from build123d import *

# Parameters (mm, degrees)
BOSS_EXTRUDE1_DEPTH = 3
BOSS_EXTRUDE2_DEPTH = 0.63
FILLET1_R           = 0.5


with BuildPart() as part:
    # Sketch1 → Boss-Extrude1 (new body)
    with BuildSketch(Plane.XY):
        with BuildLine():
            Line((-3.5, 18.4), (-2.5, 18.4))
            ThreePointArc((-2.5, 18.4), (-1.863603897, 18.663603897), (-1.6, 19.3))
            Line((-1.6, 19.3), (-1.6, 22.8))
            ThreePointArc((-1.6, 22.8), (-1.863603897, 23.436396103), (-2.5, 23.7))
            Line((-2.5, 23.7), (-3.5, 23.7))
            ThreePointArc((-3.5, 23.7), (-4.136396103, 23.436396103), (-4.4, 22.8))
            Line((-4.4, 22.8), (-4.4, 19.3))
            ThreePointArc((-4.4, 19.3), (-4.136396103, 18.663603897), (-3.5, 18.4))
        make_face()
    extrude(amount=-BOSS_EXTRUDE1_DEPTH)

    # Sketch2 → Boss-Extrude2 (add)
    with BuildSketch(Plane.XY):
        with BuildLine():
            Line((-3.5, 17.4), (-2.5, 17.4))
            ThreePointArc((-2.5, 17.4), (-1.156497116, 17.956497116), (-0.6, 19.3))
            Line((-0.6, 19.3), (-0.6, 22.8))
            ThreePointArc((-0.6, 22.8), (-1.156497116, 24.143502884), (-2.5, 24.7))
            Line((-2.5, 24.7), (-3.5, 24.7))
            ThreePointArc((-3.5, 24.7), (-4.843502884, 24.143502884), (-5.4, 22.8))
            Line((-5.4, 22.8), (-5.4, 19.3))
            ThreePointArc((-5.4, 19.3), (-4.843502884, 17.956497116), (-3.5, 17.4))
        make_face()
    extrude(amount=BOSS_EXTRUDE2_DEPTH)

    # Fillet1
    fillet1_edges = [part.edges().sort_by_distance(p)[0] for p in [
        (-3, 18.4, -3),
        (-1.863603897, 18.663603897, -3),
        (-1.6, 21.05, -3),
        (-1.863603897, 23.436396103, -3),
        (-3, 23.7, -3),
        (-4.136396103, 23.436396103, -3),
        (-4.4, 21.05, -3),
        (-4.136396103, 18.663603897, -3),
    ]]
    fillet(fillet1_edges, radius=FILLET1_R)


solid = part.part
The model under review builds one solid part; all positions refer to its coordinate system, in mm. A direction names the side the tool comes from. Round coordinates to 2 decimals unless told otherwise and drop trailing zeros. Order: outer loops, then holes, each group sorted by start corner. A loop starts at its lowest first (then second) coordinate and runs counter-clockwise, first axis right, second up. Notation, with made-up numbers: (-34.5, 12.5) - (6.5, 12.5) arc R36 ccw to (6.5, 49.5) - close; hole circle Ø2 at (-15, 60.5). An arc over 180 degrees is marked (long way). Use one line per item in the form item = value.
Q1. Tool access review of faces 1 (the cylindrical face through (-1.87, 18.66, -1.23)), 2 (the cylindrical face through (-4.14, 18.67, -1.23)), 3 (the cylindrical face through (-1.86, 23.43, -1.23)), 4 (the flat face through (-3, 18.4, -1)): name each direction out of +Z, -Z, +X, -X, +Y, -Y from which nothing blocks a thin tool from reaching the whole face with its end or side.
Response values:
face_1 = -Z, +X, -Y
face_2 = -Z, -X, -Y
face_3 = -Z, +X, +Y
face_4 = -Z, +X, -X, -Y
Q2. Add section D-D on z = -1. Give the boundary of the cut face in (x, y).
Response values:
outline = (-4.4, 19.3) arc R0.9 ccw to (-3.5, 18.4) - (-2.5, 18.4) arc R0.9 ccw to (-1.6, 19.3) - (-1.6, 22.8) arc R0.9 ccw to (-2.5, 23.7) - (-3.5, 23.7) arc R0.9 ccw to (-4.4, 22.8) - close
Q3. Add section B-B on x = -3.1. Give the boundary of the cut face in (y, z).
Response values:
outline = (17.4, 0) - (18.4, 0) - (18.4, -2.5) arc R0.5 ccw to (18.9, -3) - (23.2, -3) arc R0.5 ccw to (23.7, -2.5) - (23.7, 0) - (24.7, 0) - (24.7, 0.63) - (17.4, 0.63) - close
Q4. Add section C-C on y = 19.75. Give the boundary of the cut face in (x, z), then the cut area to 3 significant figures.
Response values:
outline = (-5.4, 0) - (-4.4, 0) - (-4.4, -2.5) arc R0.5 ccw to (-3.9, -3) - (-2.1, -3) arc R0.5 ccw to (-1.6, -2.5) - (-1.6, 0) - (-0.6, 0) - (-0.6, 0.63) - (-5.4, 0.63) - close
area = 11.3 mm^2
Q5. To check wall thickness, follow line 1 (Z direction, x = -5.1, y = 20.25); line 2 (Y direction, x = -3.05, z = -2.05); line 3 (X direction, y = 22, z = -1.45). State the ranges of each line that lie inside material, in increasing order.
Response values:
line_1 = 0 to 0.63
line_2 = 18.4 to 23.7
line_3 = -4.4 to -1.6
Q6. Add section A-A on z = 0.35. Give the boundary of the cut face in (x, y).
Response values:
outline = (-5.4, 19.3) arc R1.9 ccw to (-3.5, 17.4) - (-2.5, 17.4) arc R1.9 ccw to (-0.6, 19.3) - (-0.6, 22.8) arc R1.9 ccw to (-2.5, 24.7) - (-3.5, 24.7) arc R1.9 ccw to (-5.4, 22.8) - close
Q7. Clearance check with flat-ended pins moving along their axes: P1, Ø2, axis at y = 22, z = -1.5, coming from the +X side; P2, Ø0.8, axis at y = 21.5, z = -1.5, coming from the -X side; P3, Ø0.8, axis at x = -3, z = -1, coming from the +Y side. State where each tip first meets the part, or that it passes through.
Response values:
P1 = -1.6
P2 = -4.4
P3 = 23.7
